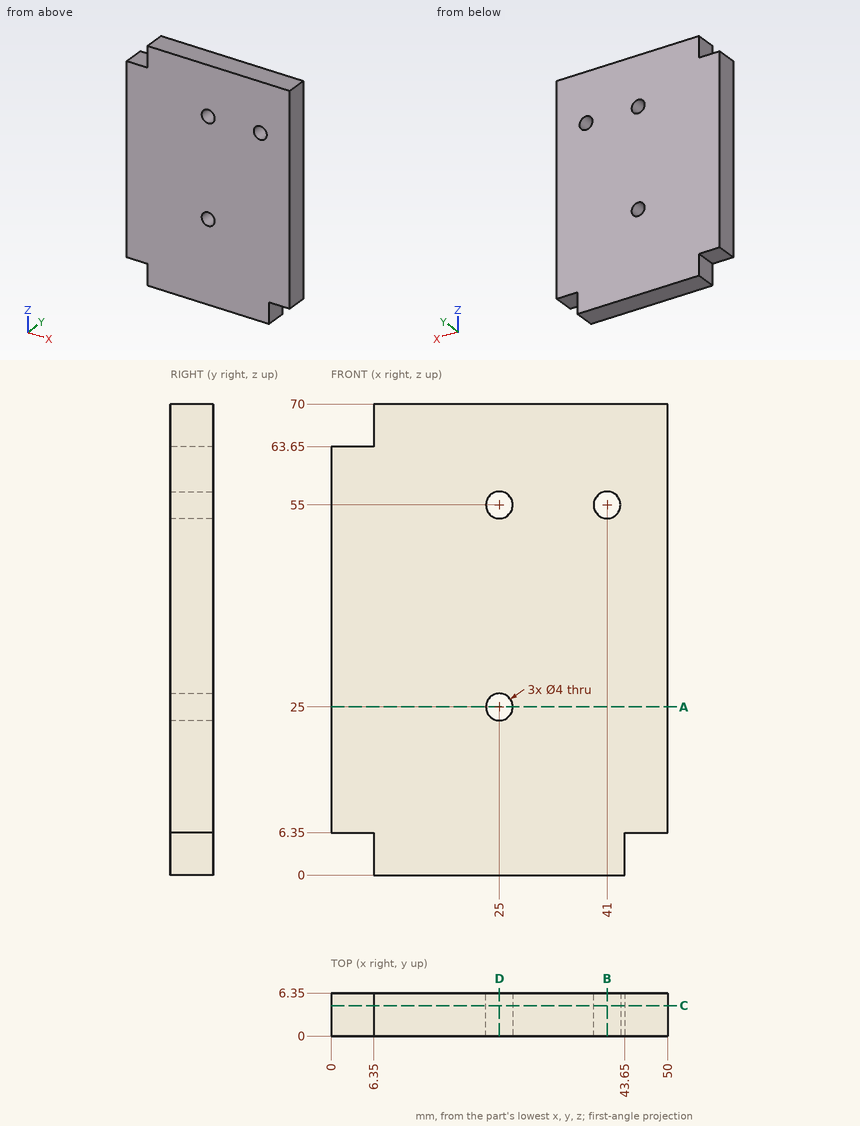
The drawing under review shows one solid part. Ordinate dimensions are in mm from its lowest x, y, z. Coordinates: 2 decimals unless noted, no trailing zeros. Loops run counter-clockwise (first coordinate to the right, second up) from the corner with the lowest first, then second, coordinate; pieces in that order, holes last.
Item 1: Add section B-B (x = 41). Write out the cut boundary in (y, z).
Completed:
outline: (0, 0) - (6.35, 0) - (6.35, 53) - (0, 53) - close; (0, 57) - (6.35, 57) - (6.35, 70) - (0, 70) - close
Item 2: Wall thickness on L1, parallel to Z at x = 25, y = 3.5; L2, parallel to Z at x = 41, y = 3.75; L3, parallel to X at y = 1.75, z = 54: over which ranges is each line inside the solid? List them lowest first.
Completed:
L1: z = 0 to 23, 27 to 53, 57 to 70
L2: z = 0 to 53, 57 to 70
L3: x = 0 to 23.27, 26.73 to 39.27, 42.73 to 50
Item 3: Add section C-C (y = 4.5). Write out the cut boundary in (x, z), and give its area (3 significant figures).
Completed:
outline: (0, 6.35) - (6.35, 6.35) - (6.35, 0) - (43.65, 0) - (43.65, 6.35) - (50, 6.35) - (50, 70) - (6.35, 70) - (6.35, 63.65) - (0, 63.65) - close; hole circle Ø4 at (25, 25); hole circle Ø4 at (25, 55); hole circle Ø4 at (41, 55)
area: 3,340 mm2
Item 4: Add section A-A (z = 25). Write out the cut boundary in (x, y).
Completed:
outline: (0, 0) - (23, 0) - (23, 6.35) - (0, 6.35) - close; (27, 0) - (50, 0) - (50, 6.35) - (27, 6.35) - close
Item 5: Add section D-D (x = 25). Write out the cut boundary in (y, z).
Completed:
outline: (0, 0) - (6.35, 0) - (6.35, 23) - (0, 23) - close; (0, 27) - (6.35, 27) - (6.35, 53) - (0, 53) - close; (0, 57) - (6.35, 57) - (6.35, 70) - (0, 70) - close
